Read the model definition and answer for the solid it produces. Units are mm, in the model's axes. A direction names the side the tool comes from. Coordinates: 2 decimals unless noted, no trailing zeros. Write each loop counter-clockwise with the first axis right and the second up, starting at its lowest first coordinate (ties: lowest second). Pieces come first, ordered by that corner, then holes. Notation, with made-up numbers: (58, -27.5) - (80, -27.5) arc R18 ccw to (80, -23.5) - close; hole circle Ø10 at (50, 75.5). An arc over 180 degrees is marked (long way). Use a Markdown table: item, result.
from build123d import *

# Parameters (mm, degrees)
F0_W     = 13
F0_H     = 13
F1_DEPTH = 110
F2_W     = 80
F2_H     = 6.5
F3_DEPTH = 5


# Not quite as in the source:
# - a pattern or mirror of a feature is missing from the dataset's text; its kind, count and spacing are read off the source's solid


with BuildPart() as f1:
    # F0 (on Right) → F1 (new body)
    with BuildSketch(Plane.YZ):
        Rectangle(F0_W, F0_H)
    extrude(amount=F1_DEPTH)

    # F2 (on face) → F3 (cut)
    with BuildSketch(Plane.XZ.offset(6.5)):
        with Locations((69.8135038838, -0.0667710053)):
            Rectangle(F2_W, F2_H)
    f3 = extrude(amount=-F3_DEPTH, mode=Mode.SUBTRACT)

    # F3_copies: F3 across plane
    add(f3.mirror(Plane.ZX), mode=Mode.SUBTRACT)


solid = f1.part
(1) The mould has two halves that part along X. Classify faces 4 (the flat face through (0, 0, 0)), 5 (the flat face through (109.814, -4, 0)), 6 (the flat face through (54, 0, -6.5)): pulls with the +X half, pulls with the -X half, needs draft (parallel to the pull), parting line crosses it, or undercut.
Report:
| item | result |
|---|---|
| face 4 | pulls with the -X half |
| face 5 | undercut |
| face 6 | needs draft |
(2) Each of these flat-tipped pins is pushed along its axis until it touches: P1, Ø5, axis at x = 88, z = 0.5, coming from the -Y side; P2, Ø4, axis at x = 59, z = 1, coming from the +Y side. Where does it stop, or does it pass through?
Report:
| item | result |
|---|---|
| P1 | stops at y = -1.5 |
| P2 | stops at y = 1.5 |
(3) A cutting plane is placed at C-C, the plane x = 61.5. Write down the section's boundary in (y, z).
Report:
| item | result |
|---|---|
| outline | (-6.5, -6.5) - (6.5, -6.5) - (6.5, -3.32) - (1.5, -3.32) - (1.5, 3.18) - (6.5, 3.18) - (6.5, 6.5) - (-6.5, 6.5) - (-6.5, 3.18) - (-1.5, 3.18) - (-1.5, -3.32) - (-6.5, -3.32) - close |
(4) For faces 1 (the flat face through (54, 0, 6.5)), 2 (the flat face through (69, 1.5, 0)), 3 (the flat face through (69, -4, 3.183)), determine the directions among +Z, -Z, +X, -X, +Y, -Y from which every point of the face is accessible in a straight line to the end or side of a thin tool.
Report:
| item | result |
|---|---|
| face 1 | +Z, +X, -X, +Y, -Y |
| face 2 | +Y |
| face 3 | -Y |
(5) A cutting plane is placed at A-A, the plane y = 5. Write down the section's boundary in (x, z).
Report:
| item | result |
|---|---|
| outline | (0, -6.5) - (110, -6.5) - (110, 6.5) - (0, 6.5) - close; hole (29.81, -3.32) - (109.81, -3.32) - (109.81, 3.18) - (29.81, 3.18) - close |
(6) Straight lines are drawn through the part: L1, parallel to Z at x = 79, y = 5.75; L2, parallel to X at y = -3.25, z = 2; L3, parallel to Y at x = 99, z = -2.25. For each, find the intervals that lie inside material, in ascending order.
Report:
| item | result |
|---|---|
| L1 | z = -6.5 to -3.32, 3.18 to 6.5 |
| L2 | x = 0 to 29.81, 109.81 to 110 |
| L3 | y = -1.5 to 1.5 |
(7) A cutting plane is placed at B-B, the plane z = -1.75. Write down the section's boundary in (x, y), and give its area (3 significant figures).
Report:
| item | result |
|---|---|
| outline | (0, -6.5) - (29.81, -6.5) - (29.81, -1.5) - (109.81, -1.5) - (109.81, -6.5) - (110, -6.5) - (110, 6.5) - (109.81, 6.5) - (109.81, 1.5) - (29.81, 1.5) - (29.81, 6.5) - (0, 6.5) - close |
| area | 630 mm² |
